Source: CAD feature listing. Evaluate the final solid. Frame: model axes, mm. A direction names the side the tool comes from. Round coordinates to 2 decimals unless told otherwise and drop trailing zeros. Order: outer loops, then holes, each group sorted by start corner. A loop starts at its lowest first (then second) coordinate and runs counter-clockwise, first axis right, second up. Notation, with made-up numbers: (78.5, -19.5) - (111.5, -19.5) arc R29 cw to (111.5, 9.5) - close; hole circle Ø7 at (23, 48.5). An arc over 180 degrees is marked (long way). Put each result on its own line as item: value. Start each with the question number.
1) Section C-C on y = 29.5. Output: boundary loops of the cut face in (x, z), then the cut area to 3 significant figures.
2) Line query: probe 1 along X at (y, z) = (13.5, 119); probe 2 along X at (y, z) = (8.5, 902). Output: solid intervals per line, ascending. Write a range as [from, to].
3) Section A-A on z = 410. Output: boundary loops of the cut face in (x, y), then the cut area to 3 significant figures.
4) Access query for faces 1 (the face through (4.762, 23, 620)), 2 (the face through (19, 0, 620)). Directions: +Z, -Z, +X, -X, +Y, -Y. A direction counts if a zero-diameter tool reaches every point of the face in a straight line with its end or side. Return the directions, or none.
5) Contact query for flat-ended pins moving along their axis: P1, Ø8, axis at y = 29, z = 528, coming from the +X side; P2, Ø10, axis at x = 18.5, z = 1057.5, coming from the -Y side; P3, Ø8, axis at x = 25, y = 6, coming from the -Z side; P4, Ø10, axis at x = 14, z = 503, coming from the +Y side. Output: stop coordinate, or through.
6) Section B-B on x = 24. Output: boundary loops of the cut face in (y, z), then the cut area to 3 significant figures.
Autodesk Inventor part; units mm, degrees
ref_plane "Start plane" through (0, 0, 0) normal (0, 0, 1) x (1, 0, 0)
ref_plane "End plane" through (0, 0, 1257.3) normal (0, 0, 1) x (1, 0, 0)
ref_plane "Work Plane4" through (19.05, 0, 1257.3) normal (0, 0.7071, 0.7071) x (1, 0, 0)
ref_plane "Start plane" through (0, 0, 0) normal (0, 0, 1) x (1, 0, 0)
ref_plane "End plane" through (0, 0, 1257.3) normal (0, 0, 1) x (1, 0, 0)
sketch "Sketch" plane through (0, 0, 0) normal (0, 0, 1) x (1, 0, 0)
  line L0 (38.1, 0) -> (0, 0)
  line L1 (0, 0) -> (0, 38.1)
  line L2 (0, 38.1) -> (2.4765, 38.1)
  line L3 (4.7625, 35.814) -> (4.7625, 9.5885)
  line L4 (9.5885, 4.7625) -> (35.814, 4.7625)
  line L5 (38.1, 2.4765) -> (38.1, 0)
  line L6 (0, -11.0414) -> (0, 31.5385) construction
  line L7 (-11.0414, 0) -> (31.5385, 0) construction
  arc A0 (4.7625, 9.5885) -> (9.5885, 4.7625) centre (9.5885, 9.5885) ccw
  arc A1 (4.7625, 35.814) -> (2.4765, 38.1) centre (2.4765, 35.814) ccw
  arc A2 (38.1, 2.4765) -> (35.814, 4.7625) centre (35.814, 2.4765) ccw
  line L8 (0, 48.4964) -> (0, -20.9644) construction
  line L9 (-20.9644, 0) -> (48.4964, 0) construction
  point P0 (4.7625, 38.1)
  point P1 (4.7625, 4.7625)
  point P2 (38.1, 4.7625)
  dimension "d0" = 38.1
  dimension "d1" = 38.1
  dimension "d2" = 4.7625
  dimension "d3" = 4.7625
  dimension "d10" = 0
  dimension "d11" = 0
  dimension "d14" = 4.826
  dimension "d15" = 2.286
extrude "Body" add sketch "Sketch" along normal up to surface (1257.3 mm away) from surface at 0
sketch "Sketch3" plane through (0, 0, 0) normal (0, 0, 1) x (1, 0, 0)
  line L0 (0, 0) -> (10, 0)
ref_plane "Work Plane3" through (0, 0, 0) normal (0, -1, 0) x (1, 0, 0)
sketch "Sketch4" plane through (0, 0, 0) normal (0, -1, 0) x (1, 0, 0)
  line L0 (-2, 0) -> (12, 0)
  line L1 (-2, 1257.3) -> (12, 1257.3)
  dimension "d17" = 1257.3
ref_plane "Work Plane4" through (19.05, 0, 1257.3) normal (0, 0.7071, 0.7071) x (1, 0, 0)
split "Split1" plane through (19.05, 0, 1257.3) removes the side toward (0, 0.7071, 0.7071)
ref_plane "Work Plane5" through (19.05, 0, 0) normal (0, 0.7071, -0.7071) x (1, 0, 0)
split "Split2" plane through (19.05, 0, 0) removes the side toward (0, 0.7071, -0.7071)
equation "\"d0\" = G_H"
equation "\"d1\" = G_H"
equation "\"d2\" = G_T"
equation "\"d3\" = G_T"
equation "\"d14\" = G_IR"
equation "\"d15\" = G_ER"
equation "\"d4\" = G_L"
equation "\"G_H\" = 38.1"
equation "\"G_T\" = 4.7625"
equation "\"G_ER\" = 2.286"
equation "\"G_IR\" = 4.826"
equation "\"G_L\" = d17"
equation "\"ex\" = 0"
equation "\"G_OFFSET_START\" = 0"
equation "\"G_OFFSET_END\" = 0"
equation "\"d13\" = G_OFFSET_END + B_L"
equation "\"B_L\" = 1257.3"
properties part number "AISC - L 1.5 x 1.5 x 3/16 - 49.5" material "Aluminum 6061-AHC"
Answer sheet:
1. outline: (0, 29.5) - (4.76, 29.5) - (4.76, 1227.8) - (0, 1227.8) - close
1. area: 5,710 mm^2
2. probe 1: [0, 4.76]
2. probe 2: [0, 4.89]
3. outline: (0, 0) - (38.1, 0) - (38.1, 2.48) arc R2.29 ccw to (35.81, 4.76) - (9.59, 4.76) arc R4.83 cw to (4.76, 9.59) - (4.76, 35.81) arc R2.29 ccw to (2.48, 38.1) - (0, 38.1) - close
3. area: 343 mm^2
4. face 1: +Z, -Z, +X, +Y
4. face 2: +Z, -Z, +X, -X, -Y
5. P1: x = 4.76
5. P2: y = 0
5. P3: z = 2
5. P4: y = 4.8
6. outline: (0, 0) - (4.76, 4.76) - (4.76, 1252.54) - (0, 1257.3) - close
6. area: 5,970 mm^2
